```python
from build123d import *

# Parameters (mm, degrees)
F0_R     = 4.9
F0_R_2   = 46
F1_DEPTH = 10


with BuildPart() as f1:
    # F0 (on Top) → F1 (new body)
    with BuildSketch(Plane.XY):
        with BuildLine():
            Line((1.389526, 78.987779), (-30.005897, 64.347853))
            ThreePointArc((-30.005897, 64.347853), (-64.347853, -30.005897), (30.005897, -64.347853))
            Line((30.005897, -64.347853), (61.401319, -49.707927))
            ThreePointArc((61.401319, -49.707927), (71.598315, 33.386843), (1.389526, 78.987779))
        make_face()
        with Locations((-28.60465, -49.544707)):
            Circle(F0_R, mode=Mode.SUBTRACT)
        with Locations((-57.2093, 0)):
            Circle(F0_R, mode=Mode.SUBTRACT)
        Circle(F0_R_2, mode=Mode.SUBTRACT)
        with Locations((28.60465, -49.544707)):
            Circle(F0_R, mode=Mode.SUBTRACT)
        with Locations((57.2093, 0)):
            Circle(F0_R, mode=Mode.SUBTRACT)
        with Locations((-28.60465, 49.544707)):
            Circle(F0_R, mode=Mode.SUBTRACT)
        with Locations((28.60465, 49.544707)):
            Circle(F0_R, mode=Mode.SUBTRACT)
    extrude(amount=F1_DEPTH)


solid = f1.part
```
Geometry: final body of the model. Coordinates: model frame, mm. Round coordinates to 2 decimals unless told otherwise and drop trailing zeros. Write each loop counter-clockwise with the first axis right and the second up, starting at its lowest first coordinate (ties: lowest second). Pieces come first, ordered by that corner, then holes. Notation, with made-up numbers: M 74.25,65 L 96.25,65 A27 cw 96.25,101 Z; hole C 5,17.5 d4. An arc over 180 degrees is marked long. Answer in a Markdown table with one row per item. Add a question column.
(1) Draft query along X for faces 1 (the face through (52.314, 0.215, 4.93)), 2 (the face through (72.112, 32.263, 4.93)), 3 (the face through (-14.09, 71.77, 4.93)), 4 (the face through (36, 38, 10)). Return one class per face: pulls with the +X half, pulls with the -X half, needs draft (parallel to the pull), parting line crosses it, or undercut.
(2) Cut plane A-A, the plane y = 0. Return the cut outline in (x, z).
(3) Cut plane B-B, the plane x = 40.5. Return the cut outline in (y, z), then the cut area to 3 significant figures.
(4) Cut plane C-C, the plane z = 5.25. Return the cut outline in (x, y).
(5) Contact query for flat-ended pins moving along their axis: pin 1 (2 mm diameter, centred on y = 48, z = 5.5, fed in from +X); pin 2 (6 mm diameter, centred on x = 28.6, y = -49.54, fed in from +Z); pin 3 (5 mm diameter, centred on x = 26.5, z = 6, fed in from -Y); pin 4 (1.5 mm diameter, centred on x = -51, z = 7.5, fed in from -Y). Output: stop coordinate, or through.
(6) Ray query, L1, parallel to Y at x = -24.5, z = 4.75; L2, parallel to X at y = -52, z = 5; L3, parallel to X at y = -54, z = 8.75. Return the intervals inside material, ascending.
(7) Cut plane D-D, the plane x = 9. Return the cut outline in (y, z).
Established:
| question | item | result |
|---|---|---|
| 1 | face 1 | undercut |
| 1 | face 2 | pulls with the +X half |
| 1 | face 3 | pulls with the -X half |
| 1 | face 4 | needs draft |
| 2 | outline | M -71,0 L -62.11,0 L -62.11,10 L -71,10 Z; M -52.31,0 L -46,0 L -46,10 L -52.31,10 Z; M 46,0 L 52.31,0 L 52.31,10 L 46,10 Z; M 62.11,0 L 79,0 L 79,10 L 62.11,10 Z |
| 3 | outline | M -59.45,0 L -21.81,0 L -21.81,10 L -59.45,10 Z; M 21.81,0 L 67.83,0 L 67.83,10 L 21.81,10 Z |
| 3 | area | 837 mm² |
| 4 | outline | M -30.01,64.35 A71 ccw 30.01,-64.35 L 61.4,-49.71 A79 ccw 1.39,78.99 Z; hole C -57.21,0 d9.8; hole C 0,0 d92; hole C -28.6,-49.54 d9.8; hole C -28.6,49.54 d9.8; hole C 28.6,-49.54 d9.8; hole C 28.6,49.54 d9.8; hole C 57.21,0 d9.8 |
| 5 | pin 1 | x = 63.5 |
| 5 | pin 2 | through |
| 5 | pin 3 | y = -66.82 |
| 5 | pin 4 | y = -50.16 |
| 6 | L1 | -66.64 to -52.22, -46.87 to -38.93, 38.93 to 46.87, 52.22 to 66.92 |
| 6 | L2 | -48.34 to -32.85, -24.36 to 24.36, 32.85 to 56.49 |
| 6 | L3 | -46.1 to -30.64, -26.56 to 26.56, 30.64 to 52.2 |
| 7 | outline | M -70.43,0 L -45.11,0 L -45.11,10 L -70.43,10 Z; M 45.11,0 L 78.49,0 L 78.49,10 L 45.11,10 Z |
